Model file for the job. Use its own axes, mm. A direction names the side the tool comes from. Round coordinates to 2 decimals unless told otherwise and drop trailing zeros. Order: outer loops, then holes, each group sorted by start corner. A loop starts at its lowest first (then second) coordinate and runs counter-clockwise, first axis right, second up. Notation, with made-up numbers: (-4, 53) - (40, 53) arc R10 ccw to (40, 64) - close; hole circle Ø9 at (53.25, 78.25). An arc over 180 degrees is marked (long way). Put each result on its own line as item: value. Start each with the question number.
Item 1: Probe probe 1 along Z at (x, y) = (70, -543.5); probe 2 along X at (y, z) = (-458, -114.5); probe 3 along Y at (x, z) = (-58.5, 273). List the from-to ranges inside material, lowest first.
Item 2: Pin check, flat tips, straight feed: pin 1 Ø4 at (x, z) = (-113.5, 71.5) entering from -Y; pin 2 Ø8 at (x, y) = (-115, -516.5) entering from +Z; pin 3 Ø6 at (y, z) = (-593.5, -70.5) entering from -X. Stop position of each tip, or through.
Item 3: Saw through at B-B on y = -407.5. List the corners of the cut face in (x, z), plus the area to 3 significant figures.
Item 4: Which spindle directions (+Z, -Z, +X, -X, +Y, -Y) get a long thin tool onto all of the face, cutting with end or side? Do faces 1 (the face through (-3, -152.4, 231)), 2 (the face through (-3, 0, 5)). Say none if no direction does.
Item 5: Saw through at D-D on z = 177.5. List the corners of the cut face in (x, y), plus the area to 3 significant figures.
Item 6: Saw through at C-C on x = 89. List the corners of the cut face in (y, z), plus the area to 3 significant figures.
Item 7: Saw through at A-A on z = -233. List the corners of the cut face in (x, y).
```python
from build123d import *

# Parameters (mm, degrees)
F0_W        = 457.2
F0_H        = 762
F1_DEPTH    = 762
F2_W        = 457.2
F2_H        = 304.8
F3_DEPTH    = 609.6
F4_T1_DEPTH = 1981.2


# Not quite as in the source:
# - a fillet or chamfer that OpenCascade refuses, or shapes differently, is made with other operations: its cross-section is extruded or revolved along the edge and cut away or added


with BuildPart() as f1:
    # F0 (on Front) → F1 (new body)
    with BuildSketch(Plane.XZ):
        Rectangle(F0_W, F0_H)
    extrude(amount=F1_DEPTH)

    # F2 (on face) → F3 (cut)
    with BuildSketch(Plane.XZ.offset(762)):
        with Locations((0, 228.6)):
            Rectangle(F2_W, F2_H)
    extrude(amount=-F3_DEPTH, mode=Mode.SUBTRACT)

    # F4: fillet of radius 304.8 on 2 edges, made by hand

    # F4_s2 → F4_t1 (cut)
    with BuildSketch(Plane.XY.offset(-1143)):
        with BuildLine():
            ThreePointArc((-228.6, -457.2), (-139.3261469057, -672.7261469057), (76.2, -762))
            Line((76.2, -762), (-228.6, -762))
            Line((-228.6, -762), (-228.6, -457.2))
        make_face()
        with BuildLine():
            ThreePointArc((228.6, -457.2), (139.3261469057, -672.7261469057), (-76.2, -762))
            Line((-76.2, -762), (228.6, -762))
            Line((228.6, -762), (228.6, -457.2))
        make_face()
    extrude(amount=F4_T1_DEPTH, mode=Mode.SUBTRACT)


solid = f1.part
```
Results found:
1. probe 1: z = -381 to 76.2
1. probe 2: x = -228.6 to 228.6
1. probe 3: y = -152.4 to 0
2. pin 1: stops at y = -697.35
2. pin 2: stops at z = 76.2
2. pin 3: stops at x = -197.91
3. outline: (-228.6, -381) - (228.6, -381) - (228.6, 76.2) - (-228.6, 76.2) - close
3. area: 209,000 mm²
4. face 1: +Z, +X, -X, -Y
4. face 2: +Z, -Z, +X, -X, +Y
5. outline: (-228.6, -152.4) - (228.6, -152.4) - (228.6, 0) - (-228.6, 0) - close
5. area: 69,700 mm²
6. outline: (-713.35, -381) - (0, -381) - (0, 381) - (-152.4, 381) - (-152.4, 76.2) - (-713.35, 76.2) - close
6. area: 373,000 mm²
7. outline: (-228.6, -457.2) arc R304.8 ccw to (0, -752.32) arc R304.8 ccw to (228.6, -457.2) - (228.6, 0) - (-228.6, 0) - close
